Part model, mm, in its own coordinate system. Face numbers are marked on the shaded views. A direction names the side the tool comes from. Round coordinates to 2 decimals unless told otherwise and drop trailing zeros. Loops run counter-clockwise (first coordinate to the right, second up) from the corner with the lowest first, then second, coordinate; pieces in that order, holes last.
(1) Cut at D-D on x = -17. List the corners of the cut face in (y, z), then the cut area to 3 significant figures.
(2) Flat gauge pins, fed straight in: pin 1 (24 mm diameter, centred on x = 37.68, y = 51.86, fed in from -Z); pin 2 (2 mm diameter, centred on x = -52, y = 33, fed in from +Z); pin 3 (4 mm diameter, centred on y = -1.5, z = 41.5, fed in from +X). Where does each tip first touch, or does it go through?
(3) Cut at C-C on y = 0. List the corners of the cut face in (x, z).
(4) Cut at A-A on x = 0. List the corners of the cut face in (y, z).
(5) Cut at B-B on y = -61.5. List the corners of the cut face in (x, z), then the cut area to 3 significant figures.
(6) Tool access for the marked faces 1 and 2: list every direction of +Z, -Z, +X, -X, +Y, -Y with a clear straight run to the whole face (end or side of a thin tool).
(7) Probe probe 1 along Z at (x, y) = (-65, 13); probe 2 along X at (y, z) = (52, 173.5); probe 3 along Z at (x, y) = (-4, 27). List the from-to ranges inside material, lowest first.
from build123d import *

# Parameters (mm, degrees)
SKETCH1_R            = 14
BOSS_EXTRUDE2_DEPTH  = 18
BOSS_EXTRUDE7_START  = 3
SKETCH8_R            = 14
BOSS_EXTRUDE7_DEPTH  = 3
SKETCH12_R           = 14
BOSS_EXTRUDE11_DEPTH = 150
SKETCH13_R           = 7
BOSS_EXTRUDE12_DEPTH = 10
SKETCH14_R           = 78
SKETCH14_R_2         = 7.5
BOSS_EXTRUDE13_DEPTH = 10
SKETCH15_R           = 50.291796038
BOSS_EXTRUDE14_DEPTH = 10


with BuildPart() as part:
    # Sketch1 → Boss-Extrude2 (new body)
    with BuildSketch(Plane.XY):
        Circle(SKETCH1_R)
    extrude(amount=BOSS_EXTRUDE2_DEPTH)

    # Sketch8 → Boss-Extrude7 (add)
    with BuildSketch(Plane(origin=(0, 0, 0), x_dir=(-1, 0, 0), z_dir=(0, 0, -1)).offset(BOSS_EXTRUDE7_START)):
        Circle(SKETCH8_R)
    extrude(amount=-BOSS_EXTRUDE7_DEPTH)

    # Sketch12 → Boss-Extrude11 (add)
    with BuildSketch(Plane.XY.offset(18)):
        with Locations(Location((0, 0, 0), (0, 0, 180))):
            Circle(SKETCH12_R)
    extrude(amount=BOSS_EXTRUDE11_DEPTH)

    # Sketch13 → Boss-Extrude12 (add)
    with BuildSketch(Plane(origin=(0, 0, -3), x_dir=(-1, 0, 0), z_dir=(0, 0, -1))):
        Circle(SKETCH13_R)
    extrude(amount=BOSS_EXTRUDE12_DEPTH)

    # Sketch14 → Boss-Extrude13 (add)
    with BuildSketch(Plane.XY.offset(168)):
        Circle(SKETCH14_R)
        with Locations((0, -64.10766693)):
            Circle(SKETCH14_R_2, mode=Mode.SUBTRACT)
        with Locations((-60.970014378, -19.810358551)):
            Circle(SKETCH14_R_2, mode=Mode.SUBTRACT)
        with Locations((-37.68154118, 51.864192016)):
            Circle(SKETCH14_R_2, mode=Mode.SUBTRACT)
        with Locations((37.68154118, 51.864192016)):
            Circle(SKETCH14_R_2, mode=Mode.SUBTRACT)
        with Locations((60.970014378, -19.810358551)):
            Circle(SKETCH14_R_2, mode=Mode.SUBTRACT)
    extrude(amount=BOSS_EXTRUDE13_DEPTH)

    # Sketch15 → Boss-Extrude14 (add)
    with BuildSketch(Plane.XY.offset(178)):
        Circle(SKETCH15_R)
    extrude(amount=BOSS_EXTRUDE14_DEPTH)


solid = part.part
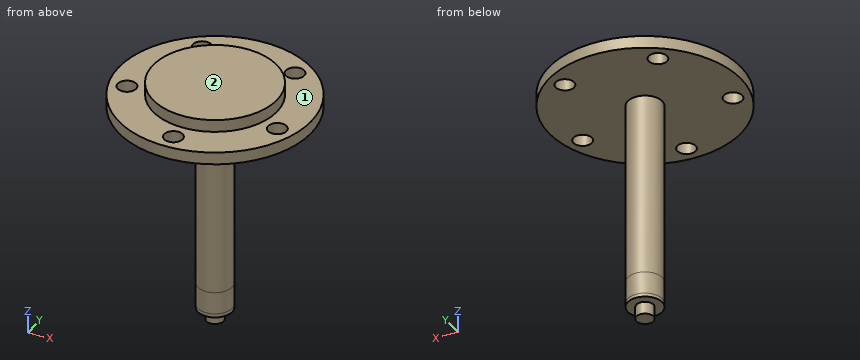
Final values:
1. outline: (-76.12, 168) - (76.12, 168) - (76.12, 178) - (47.33, 178) - (47.33, 188) - (-47.33, 188) - (-47.33, 178) - (-76.12, 178) - close
1. area: 2,470 mm2
2. pin 1: stops at z = 168
2. pin 2: stops at z = 178
2. pin 3: stops at x = 14
3. outline: (-78, 168) - (-14, 168) - (-14, -3) - (-7, -3) - (-7, -13) - (7, -13) - (7, -3) - (14, -3) - (14, 168) - (78, 168) - (78, 178) - (50.29, 178) - (50.29, 188) - (-50.29, 188) - (-50.29, 178) - (-78, 178) - close
4. outline: (-78, 168) - (-71.61, 168) - (-71.61, 178) - (-78, 178) - close; (-56.61, 168) - (-14, 168) - (-14, -3) - (-7, -3) - (-7, -13) - (7, -13) - (7, -3) - (14, -3) - (14, 168) - (78, 168) - (78, 178) - (50.29, 178) - (50.29, 188) - (-50.29, 188) - (-50.29, 178) - (-56.61, 178) - close
5. outline: (-47.98, 168) - (-7.03, 168) - (-7.03, 178) - (-47.98, 178) - close; (7.03, 168) - (47.98, 168) - (47.98, 178) - (7.03, 178) - close
5. area: 819 mm2
6. face 1: +Z
6. face 2: +Z, +X, -X, +Y, -Y
7. probe 1: z = 168 to 178
7. probe 2: x = -58.14 to -45.18, -30.18 to 30.18, 45.18 to 58.14
7. probe 3: z = 168 to 188
